```python
from build123d import *

# Parameters (mm, degrees)
F0_R     = 25
F0_R_2   = 2.5
F1_DEPTH = 6


with BuildPart() as f1:
    # F0 (on Top) → F1 (new body)
    with BuildSketch(Plane.XY):
        Circle(F0_R)
        with Locations((-15.974261, -10.287031)):
            Circle(F0_R_2, mode=Mode.SUBTRACT)
        with Locations((16.89596, -8.6906)):
            Circle(F0_R_2, mode=Mode.SUBTRACT)
        with BuildLine():
            ThreePointArc((0, 7), (4.949747, 4.949747), (7, 0))
            ThreePointArc((7, 0), (-4.949747, -4.949747), (0, 7))
        make_face(mode=Mode.SUBTRACT)
        with BuildLine():
            ThreePointArc((2.5, 19), (1.767767, 17.232233), (0, 16.5))
            ThreePointArc((0, 16.5), (-1.767767, 20.767767), (2.5, 19))
        make_face(mode=Mode.SUBTRACT)
    extrude(amount=F1_DEPTH)


solid = f1.part
```
Verification items for the finished model (mm, model axes). Coordinates: 2 decimals unless noted, no trailing zeros. Loops run counter-clockwise (first coordinate to the right, second up) from the corner with the lowest first, then second, coordinate; pieces in that order, holes last. Notation, with made-up numbers: (-14.75, 86) - (-1.75, 86) arc R28 cw to (-1.75, 110) - close; hole circle Ø9 at (-35.5, 52). An arc over 180 degrees is marked (long way). Put each result on its own line as item: value.
Item 1: Scan lines: line 1 along X through (y, z) = (-8.5, 5.05); line 2 along X through (y, z) = (-9, 5.3); line 3 along X through (y, z) = (-1, 2.7). Record each from-to range of solid material in increasing order.
Conclusion:
line 1: x = -23.51 to -17.72, -14.23 to 14.4, 19.39 to 23.51
line 2: x = -23.32 to -18.12, -13.83 to 14.42, 19.38 to 23.32
line 3: x = -24.98 to -6.93, 6.93 to 24.98
Item 2: Section check C-C (z = 2.1). Enter the section's corners in (x, y), then the cut area to 3 significant figures.
Conclusion:
outline: circle Ø50 at (0, 0); hole circle Ø5 at (-15.97, -10.29); hole circle Ø5 at (0, 19); hole (0, 7) arc R7 ccw (long way) to (7, 0) arc R7 ccw to start; hole circle Ø5 at (16.9, -8.69)
area: 1,750 mm2
Item 3: Section check D-D (y = -22). Enter the section's corners in (x, z), then the cut area to 3 significant figures.
Conclusion:
outline: (-11.87, 0) - (11.87, 0) - (11.87, 6) - (-11.87, 6) - close
area: 142 mm2
Item 4: Section check A-A (x = 4). Enter the section's corners in (y, z).
Conclusion:
outline: (-24.68, 0) - (-5.74, 0) - (-5.74, 6) - (-24.68, 6) - close; (5.74, 0) - (24.68, 0) - (24.68, 6) - (5.74, 6) - close
Item 5: Gauge pin test, flat ends, axial feed: pin 1 Ø2 at (y, z) = (4, 3.5) entering from +X; pin 2 Ø1 at (y, z) = (-15, 5) entering from -X; pin 3 Ø1 at (y, z) = (-12.5, 4) entering from +X. Record the tip position at first contact, or that the pin passes through.
Conclusion:
pin 1: stops at x = 24.82
pin 2: stops at x = -20.37
pin 3: stops at x = 21.93
Item 6: Draft check along Y on faces 1 (the face through (-18.47, -10.18, 2.96)), 2 (the face through (5.2, -5.2, 0)), 3 (the face through (23.846, 7.509, 2.958)). Enter one of: pulls with the +Y half, pulls with the -Y half, needs draft (parallel to the pull), parting line crosses it, or undercut.
Conclusion:
face 1: undercut
face 2: needs draft
face 3: parting line crosses it
